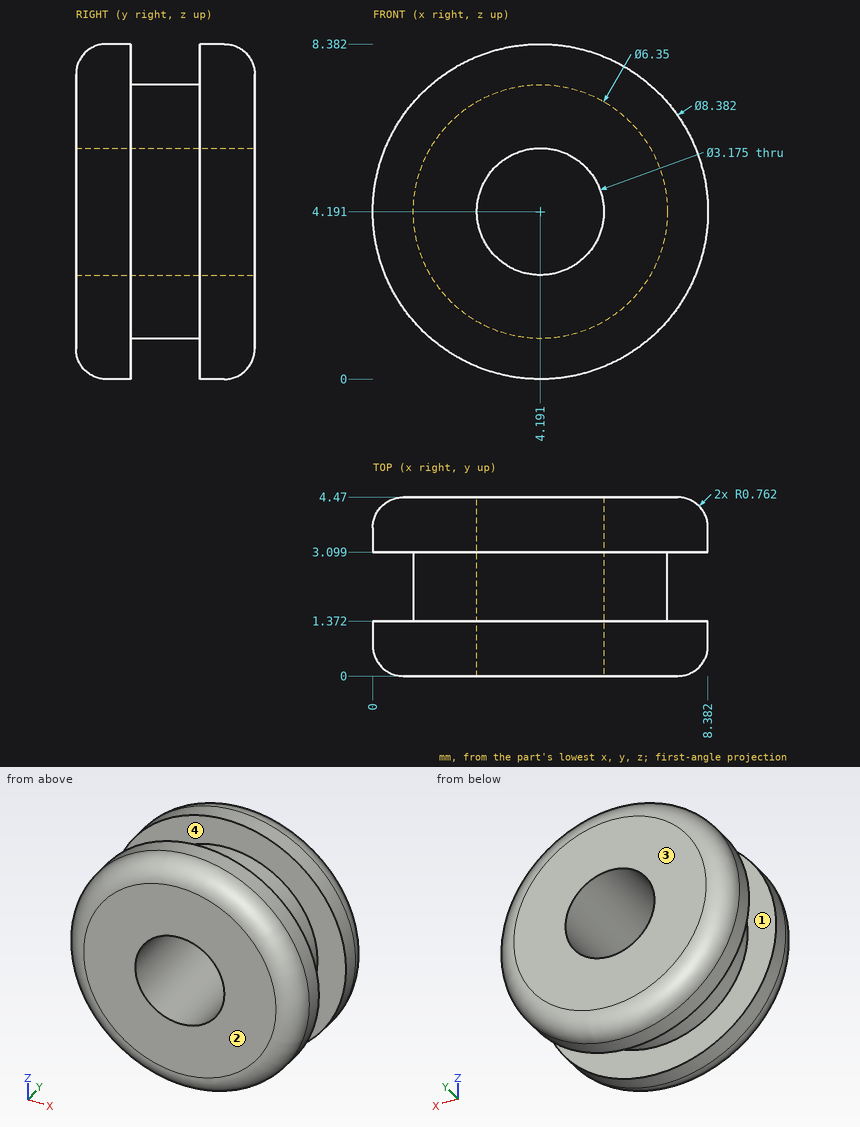
For this review, use the dimensioned drawing (mm, ordinates from the lowest corner) and the shaded views. Give positions to 0.01 mm unless a question says otherwise; leave off trailing zeros.
1. For pin 1 Ø1.5 at (y, z) = (1.5, 3) entering from -X (1 decimal); pin 2 Ø1 at (y, z) = (3.5, 7.5) entering from -X, all flat-tipped, find the tip position at first contact; note any pin that passes through.
Solution:
pin 1: stops at x = 0
pin 2: stops at x = 1.08
2. To check wall thickness, follow L1, parallel to Y at x = 3.75, z = 1; L2, parallel to X at y = 2.55, z = 3.75 (1 decimal); L3, parallel to Z at x = 4, y = 0.95 (1 decimal). State the ranges of each line that lie inside material, in increasing order.
Solution:
L1: y = 0 to 1.37, 3.1 to 4.47
L2: x = 1 to 2.7, 5.7 to 7.3
L3: z = 0 to 2.6, 5.8 to 8.4
3. Mouldability with a two-part tool opening along Y and no side actions: class the marked faces 1, 2, 3 and 4 as +Y half, -Y half, draft (parallel to the pull), parting line (faces both ways), or undercut.
Solution:
face 1: undercut
face 2: -Y half
face 3: +Y half
face 4: undercut
